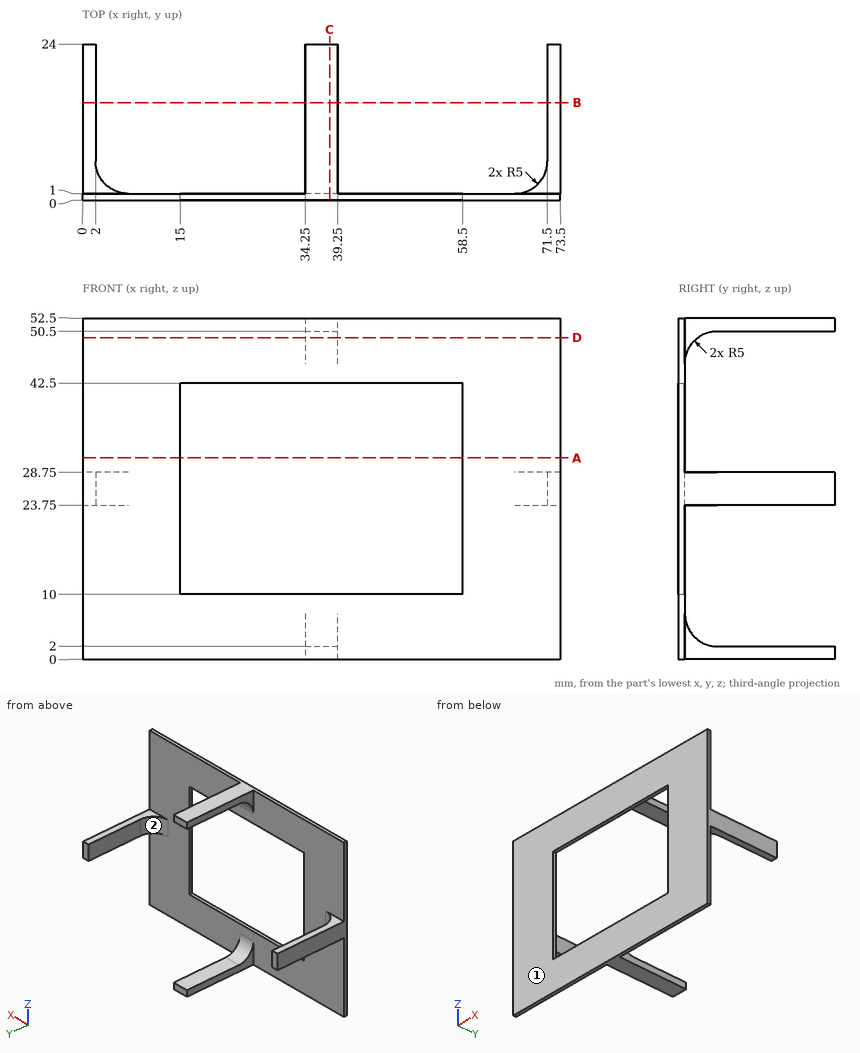
For this review, use the dimensioned drawing (mm, ordinates from the lowest corner) and the shaded views. Give positions to 0.01 mm unless a question says otherwise; leave off trailing zeros. Write each loop counter-clockwise with the first axis right and the second up, starting at its lowest first coordinate (ties: lowest second). Pieces come first, ordered by that corner, then holes.
(1) To check wall thickness, follow L1, parallel to Z at x = 36, y = 13.25; L2, parallel to Y at x = 8.5, z = 27; L3, parallel to Y at x = 34.5, z = 50. State the ranges of each line that lie inside material, in increasing order.
(2) Consider section B-B, the plane y = 15. Give the boundary of the cut face in (x, z).
(3) Consider section D-D, the plane z = 49.5. Give the boundary of the cut face in (x, y), and give its area (3 significant figures).
(4) The part is to be moulded in two halves that separate along X. For the marked faces 1 and 2, say which applies: released by +X, released by -X, zero draft, split by the parting line, or undercut.
(5) Consider section C-C, the plane x = 38. Give the boundary of the cut face in (y, z).
(6) Consider section A-A, the plane z = 31. Give the boundary of the cut face in (x, y).
(7) For P1, Ø5.5, axis at y = 8.5, z = 2, coming from the -X side; P2, Ø7.5, axis at x = 68.5, y = 18, coming from the -Z side; P3, Ø10, axis at y = 15, z = 17.5, coming from the +X side; P4, Ø3.5, axis at y = 16, z = 3, coming from the +X side, all flat-tipped, find the tip position at first contact; note any pin that passes through.
Returned:
1. L1: z = 0 to 2, 50.5 to 52.5
1. L2: y = 0 to 1
1. L3: y = 0 to 3.82
2. outline: (0, 23.75) - (2, 23.75) - (2, 28.75) - (0, 28.75) - close; (34.25, 0) - (39.25, 0) - (39.25, 2) - (34.25, 2) - close; (34.25, 50.5) - (39.25, 50.5) - (39.25, 52.5) - (34.25, 52.5) - close; (71.5, 23.75) - (73.5, 23.75) - (73.5, 28.75) - (71.5, 28.75) - close
3. outline: (0, 0) - (73.5, 0) - (73.5, 1) - (39.25, 1) - (39.25, 3) - (34.25, 3) - (34.25, 1) - (0, 1) - close
3. area: 83.5 mm2
4. face 1: zero draft
4. face 2: undercut
5. outline: (0, 0) - (24, 0) - (24, 2) - (6, 2) arc R5 cw to (1, 7) - (1, 10) - (0, 10) - close; (0, 42.5) - (1, 42.5) - (1, 45.5) arc R5 cw to (6, 50.5) - (24, 50.5) - (24, 52.5) - (0, 52.5) - close
6. outline: (0, 0) - (15, 0) - (15, 1) - (0, 1) - close; (58.5, 0) - (73.5, 0) - (73.5, 1) - (58.5, 1) - close
7. P1: stops at x = 34.25
7. P2: stops at z = 23.75
7. P3: passes through
7. P4: stops at x = 39.25
